```python
from build123d import *

# Parameters (mm, degrees)
SKETCH1_W           = 63
SKETCH1_H           = 63
BOSS_EXTRUDE1_DEPTH = 5
SKETCH2_W           = 6
SKETCH2_H           = 6
BOSS_EXTRUDE2_DEPTH = 13
SKETCH3_R           = 1.5
CUT_EXTRUDE1_DEPTH  = 5
BOSS_EXTRUDE3_START = 7.3
SKETCH4_R           = 2.7
SKETCH4_R_2         = 1.5
BOSS_EXTRUDE3_DEPTH = 7.3
BOSS_EXTRUDE4_START = 7.3
BOSS_EXTRUDE4_DEPTH = 7.3
SKETCH6_W           = 9
SKETCH6_H           = 5.4
CUT_EXTRUDE2_DEPTH  = 2.8
CUT_EXTRUDE3_REACH  = 91.94
SKETCH7_W           = 7
SKETCH7_H           = 12.7
BOSS_EXTRUDE5_START = 7.3
BOSS_EXTRUDE5_DEPTH = 7.3
SKETCH9_W           = 5.4
SKETCH9_H           = 35.5
CUT_EXTRUDE4_DEPTH  = 4.6
SKETCH10_W          = 13
SKETCH10_H          = 5.4
CUT_EXTRUDE5_DEPTH  = 4.2
SKETCH11_W          = 13
SKETCH11_H          = 5.4
CUT_EXTRUDE6_DEPTH  = 2
SKETCH12_W          = 5.4
SKETCH12_H          = 9
CUT_EXTRUDE7_DEPTH  = 2
SKETCH13_W          = 5.4
SKETCH13_H          = 6
CUT_EXTRUDE8_DEPTH  = 6
SKETCH14_W          = 3
SKETCH14_H          = 6
CUT_EXTRUDE9_DEPTH  = 4


with BuildPart() as part:
    # Sketch1 → Boss-Extrude1 (new body)
    with BuildSketch(Plane(origin=(0, 0, 0), x_dir=(1, 0, 0), z_dir=(0, 1, 0))):
        with Locations((31.5, 31.5)):
            Rectangle(SKETCH1_W, SKETCH1_H)
    extrude(amount=BOSS_EXTRUDE1_DEPTH)

    # Sketch2 → Boss-Extrude2 (add)
    with BuildSketch(Plane(origin=(0, 5, 0), x_dir=(1, 0, 0), z_dir=(0, 1, 0))):
        with Locations((3, 60)):
            Rectangle(SKETCH2_W, SKETCH2_H)
        with Locations((3, 3)):
            Rectangle(SKETCH2_W, SKETCH2_H)
        with Locations((60, 60)):
            Rectangle(SKETCH2_W, SKETCH2_H)
        with Locations((60, 3)):
            Rectangle(SKETCH2_W, SKETCH2_H)
    extrude(amount=BOSS_EXTRUDE2_DEPTH)

    # Sketch3 → Cut-Extrude1 (cut)
    with BuildSketch(Plane(origin=(0, 5, 0), x_dir=(1, 0, 0), z_dir=(0, 1, 0))):
        with Locations(Location((53, 10, 0), (0, 0, 270))):
            Circle(SKETCH3_R)
        with Locations(Location((10, 10, 0), (0, 0, 270))):
            Circle(SKETCH3_R)
        with Locations(Location((10, 53, 0), (0, 0, 270))):
            Circle(SKETCH3_R)
        with Locations(Location((53, 53, 0), (0, 0, 270))):
            Circle(SKETCH3_R)
    extrude(amount=-CUT_EXTRUDE1_DEPTH, mode=Mode.SUBTRACT)

    # Sketch4 → Boss-Extrude3 (add)
    # profile 1 of 4: a face of its own
    with BuildSketch(Plane(origin=(0, 5, 0), x_dir=(1, 0, 0), z_dir=(0, 1, 0)).offset(BOSS_EXTRUDE3_START)):
        with Locations(Location((10, 10, 0), (0, 0, 90))):
            Circle(SKETCH4_R)
        with Locations(Location((10, 10, 0), (0, 0, 270))):
            Circle(SKETCH4_R_2, mode=Mode.SUBTRACT)
    # profile 2 of 4: a face of its own
    with BuildSketch(Plane(origin=(0, 5, 0), x_dir=(1, 0, 0), z_dir=(0, 1, 0)).offset(BOSS_EXTRUDE3_START)):
        with Locations(Location((10, 53, 0), (0, 0, 90))):
            Circle(SKETCH4_R)
        with Locations(Location((10, 53, 0), (0, 0, 270))):
            Circle(SKETCH4_R_2, mode=Mode.SUBTRACT)
    # profile 3 of 4: a face of its own
    with BuildSketch(Plane(origin=(0, 5, 0), x_dir=(1, 0, 0), z_dir=(0, 1, 0)).offset(BOSS_EXTRUDE3_START)):
        with Locations(Location((53, 10, 0), (0, 0, 90))):
            Circle(SKETCH4_R)
        with Locations(Location((53, 10, 0), (0, 0, 270))):
            Circle(SKETCH4_R_2, mode=Mode.SUBTRACT)
    # profile 4 of 4: a face of its own
    with BuildSketch(Plane(origin=(0, 5, 0), x_dir=(1, 0, 0), z_dir=(0, 1, 0)).offset(BOSS_EXTRUDE3_START)):
        with Locations(Location((53, 53, 0), (0, 0, 90))):
            Circle(SKETCH4_R)
        with Locations(Location((53, 53, 0), (0, 0, 270))):
            Circle(SKETCH4_R_2, mode=Mode.SUBTRACT)
    extrude(amount=-BOSS_EXTRUDE3_DEPTH)

    # Sketch5 → Boss-Extrude4 (add)
    with BuildSketch(Plane(origin=(0, 5, 0), x_dir=(1, 0, 0), z_dir=(0, 1, 0)).offset(BOSS_EXTRUDE4_START)):
        with BuildLine():
            Line((10, 7.3), (53, 7.3))
            ThreePointArc((53, 7.3), (50.3, 10), (53, 12.7))
            Line((53, 12.7), (10, 12.7))
            ThreePointArc((10, 12.7), (12.7, 10), (10, 7.3))
        make_face()
    extrude(amount=-BOSS_EXTRUDE4_DEPTH)

    # Sketch6 → Cut-Extrude2 (cut)
    with BuildSketch(Plane(origin=(0, 12.3, 0), x_dir=(1, 0, 0), z_dir=(0, 1, 0))):
        with Locations((23, 10)):
            Rectangle(SKETCH6_W, SKETCH6_H)
    extrude(amount=-CUT_EXTRUDE2_DEPTH, mode=Mode.SUBTRACT)

    # Cut-Extrude3: up to this face of the body (flat: up to its plane)
    cut_extrude3_end = Plane(part.part.faces().sort_by_distance((31.5, 0, -31.5))[0])
    # Sketch7 → Cut-Extrude3 (cut, up to the picked face)
    with BuildSketch(Plane(origin=(0, 12.3, 0), x_dir=(1, 0, 0), z_dir=(0, 1, 0)), mode=Mode.PRIVATE) as cut_extrude3_sk1:
        with Locations((41, 6.35)):
            Rectangle(SKETCH7_W, SKETCH7_H)
    cut_extrude3_tool1 = split(extrude(cut_extrude3_sk1.sketch, amount=-CUT_EXTRUDE3_REACH, mode=Mode.PRIVATE), bisect_by=cut_extrude3_end, keep=Keep.BOTH, mode=Mode.PRIVATE)
    add(cut_extrude3_tool1.solids().sort_by(Axis((41, 12.3, -6.35), (0, -1, 0)))[0], mode=Mode.SUBTRACT)

    # Sketch8 → Boss-Extrude5 (add)
    with BuildSketch(Plane(origin=(0, 5, 0), x_dir=(1, 0, 0), z_dir=(0, 1, 0)).offset(BOSS_EXTRUDE5_START)):
        with BuildLine():
            Line((55.7, 53), (55.7, 10))
            ThreePointArc((55.7, 10), (54.909188309, 11.909188309), (53, 12.7))
            Line((53, 12.7), (50.3, 12.7))
            Line((50.3, 12.7), (50.3, 50.3))
            Line((50.3, 50.3), (12.7, 50.3))
            Line((12.7, 50.3), (12.7, 12.7))
            Line((12.7, 12.7), (10, 12.7))
            ThreePointArc((10, 12.7), (8.090811691, 11.909188309), (7.3, 10))
            Line((7.3, 10), (7.3, 53))
            ThreePointArc((7.3, 53), (8.090811691, 51.090811691), (10, 50.3))
            ThreePointArc((10, 50.3), (12.7, 53), (10, 55.7))
            Line((10, 55.7), (53, 55.7))
            ThreePointArc((53, 55.7), (51.090811691, 54.909188309), (50.3, 53))
            ThreePointArc((50.3, 53), (53, 50.3), (55.7, 53))
        make_face()
    extrude(amount=-BOSS_EXTRUDE5_DEPTH)

    # Sketch9 → Cut-Extrude4 (cut)
    with BuildSketch(Plane(origin=(0, 12.3, 0), x_dir=(1, 0, 0), z_dir=(0, 1, 0))):
        with Locations((53, 31.75)):
            Rectangle(SKETCH9_W, SKETCH9_H)
    extrude(amount=-CUT_EXTRUDE4_DEPTH, mode=Mode.SUBTRACT)

    # Sketch10 → Cut-Extrude5 (cut)
    with BuildSketch(Plane(origin=(0, 12.3, 0), x_dir=(1, 0, 0), z_dir=(0, 1, 0))):
        with Locations((42.1, 53)):
            Rectangle(SKETCH10_W, SKETCH10_H)
    extrude(amount=-CUT_EXTRUDE5_DEPTH, mode=Mode.SUBTRACT)

    # Sketch11 → Cut-Extrude6 (cut)
    with BuildSketch(Plane(origin=(0, 12.3, 0), x_dir=(1, 0, 0), z_dir=(0, 1, 0))):
        with Locations((27.1, 53)):
            Rectangle(SKETCH11_W, SKETCH11_H)
    extrude(amount=-CUT_EXTRUDE6_DEPTH, mode=Mode.SUBTRACT)

    # Sketch12 → Cut-Extrude7 (cut)
    with BuildSketch(Plane(origin=(0, 12.3, 0), x_dir=(1, 0, 0), z_dir=(0, 1, 0))):
        with Locations((10, 37.5)):
            Rectangle(SKETCH12_W, SKETCH12_H)
    extrude(amount=-CUT_EXTRUDE7_DEPTH, mode=Mode.SUBTRACT)

    # Sketch13 → Cut-Extrude8 (cut)
    with BuildSketch(Plane(origin=(0, 12.3, 0), x_dir=(1, 0, 0), z_dir=(0, 1, 0))):
        with Locations((10, 22)):
            Rectangle(SKETCH13_W, SKETCH13_H)
    extrude(amount=-CUT_EXTRUDE8_DEPTH, mode=Mode.SUBTRACT)

    # Sketch14 → Cut-Extrude9 (cut)
    with BuildSketch(Plane(origin=(0, 18, 0), x_dir=(1, 0, 0), z_dir=(0, 1, 0))):
        with Locations((1.5, 3)):
            Rectangle(SKETCH14_W, SKETCH14_H)
        with Locations((61.5, 3)):
            Rectangle(SKETCH14_W, SKETCH14_H)
        with Locations((61.5, 60)):
            Rectangle(SKETCH14_W, SKETCH14_H)
        with Locations((1.5, 60)):
            Rectangle(SKETCH14_W, SKETCH14_H)
    extrude(amount=-CUT_EXTRUDE9_DEPTH, mode=Mode.SUBTRACT)


solid = part.part
```
Can you work these out from the model? Positions are in its coordinate system, mm. A direction names the side the tool comes from. Coordinates: 2 decimals unless noted, no trailing zeros. Loops run counter-clockwise (first coordinate to the right, second up) from the corner with the lowest first, then second, coordinate; pieces in that order, holes last. Notation, with made-up numbers: (-21.75, 67) - (2.25, 67) arc R32 cw to (2.25, 93) - close; hole circle Ø1 at (59, -26). An arc over 180 degrees is marked (long way). Answer as CSV lines item,"result". Start each with the question number.
1) I need wall thicknesses on line 1 (X direction, y = 3.75, z = -53); line 2 (X direction, y = 3.75, z = -10); line 3 (X direction, y = 6.5, z = -11). Which ranges of each line are inside material? Lowest first, please. Write a range as from..to.
2) Suppose I cut it at A-A (y = 17). Please give me the cut outline in (x, z).
3) Suppose I cut it at B-B (x = 21.5). Please give me the cut outline in (y, z).
4) Suppose I cut it at D-D (z = -27). Please give me the cut outline in (x, y), plus the area to 3 significant figures.
5) Which directions (+Z, -Z, +X, -X, +Y, -Y) give clear straight access to the entire face, cutting with the end or side of a thin tool? Please do faces 5 (the flat face through (7.3, 9, -31)), 6 (the flat face through (55.7, 7, -32)), 7 (the flat face through (42, 8.1, -53)), 8 (the flat face through (6, 11, -3)).
6) Thinking about a two-plate mould opening in Z: for faces 1 (the flat face through (49, 9, -7.3)), 2 (the flat face through (53, 7.7, -32)), 3 (the cylindrical face through (54.93, 8.7, -54.89)), 4 (the flat face through (61, 14, -60)), which applies, pulls with the +Z half, pulls with the -Z half, needs draft (parallel to the pull), parting line crosses it, or undercut?
7) For pin 1 (0.9 mm diameter, centred on x = 2, z = -1.5, fed in from +Y); pin 2 (2.5 mm diameter, centred on x = 9.5, z = -36.5, fed in from +Y); pin 3 (3 mm diameter, centred on x = 54, z = -24, fed in from +Y); pin 4 (1 mm diameter, centred on x = 39, y = 12.5, fed in from +Z), each with a flat end and sliding along its axis, tell me the tip position at first contact or that it passes through.
8) Suppose I cut it at C-C (y = 2.5). Please give me the cut outline in (x, z), plus the area to 3 significant figures.
Check result:
1,line 1,"x = 0..8.5, 11.5..51.5, 54.5..63"
1,line 2,"x = 0..8.5, 11.5..37.5, 44.5..51.5, 54.5..63"
1,line 3,"x = 7.3..8.88, 11.12..37.5, 44.5..51.88, 54.12..55.7"
2,outline,"(3, -63) - (6, -63) - (6, -57) - (3, -57) - close; (3, -6) - (6, -6) - (6, 0) - (3, 0) - close; (57, -63) - (60, -63) - (60, -57) - (57, -57) - close; (57, -6) - (60, -6) - (60, 0) - (57, 0) - close"
3,outline,"(0, -63) - (5, -63) - (5, -55.7) - (10.3, -55.7) - (10.3, -50.3) - (5, -50.3) - (5, -12.7) - (9.5, -12.7) - (9.5, -7.3) - (5, -7.3) - (5, 0) - (0, 0) - close"
4,outline,"(0, 0) - (63, 0) - (63, 5) - (55.7, 5) - (55.7, 7.7) - (50.3, 7.7) - (50.3, 5) - (12.7, 5) - (12.7, 12.3) - (7.3, 12.3) - (7.3, 5) - (0, 5) - close"
4,area,"369 mm²"
5,face 5,"+Z, -Z, -X, +Y"
5,face 6,"+Z, -Z, +X, +Y"
5,face 7,"-Z, +Y"
5,face 8,"+Z, -Z, +Y"
6,face 1,"pulls with the +Z half"
6,face 2,"undercut"
6,face 3,"pulls with the -Z half"
6,face 4,"needs draft"
7,pin 1,"stops at y = 14"
7,pin 2,"stops at y = 10.3"
7,pin 3,"stops at y = 7.7"
7,pin 4,"passes through"
8,outline,"(0, -63) - (63, -63) - (63, 0) - (44.5, 0) - (44.5, -12.7) - (37.5, -12.7) - (37.5, 0) - (0, 0) - close; hole circle Ø3 at (10, -53); hole circle Ø3 at (10, -10); hole circle Ø3 at (53, -53); hole circle Ø3 at (53, -10)"
8,area,"3,850 mm²"
